Here's how the part is built. I have some questions about the finished solid (model axes, mm). A direction names the side the tool comes from. Give positions to 0.01 mm unless a question says otherwise; leave off trailing zeros. Write each loop counter-clockwise with the first axis right and the second up, starting at its lowest first coordinate (ties: lowest second). Pieces come first, ordered by that corner, then holes. Notation, with made-up numbers: (87.25, 11.25) -> (111.25, 11.25) arc R35 cw to (111.25, 50.25) -> close; hole circle Ø2 at (-26, 43). An arc over 180 degrees is marked (long way). Put each result on its own line as item: value. Start each with the question number.
from build123d import *

# Parameters (mm, degrees)
RESSALTO_EXTRUS_O1_DEPTH = 10
ESBO_O2_R                = 2.55
CORTE_EXTRUS_O1_DEPTH    = 10
ESBO_O4_R                = 19.5
CORTE_EXTRUS_O3_DEPTH    = 10
ESBO_O5_W                = 20
ESBO_O5_H                = 10
CORTE_EXTRUS_O4_DEPTH    = 30
ESBO_O6_R                = 1.75
CORTE_EXTRUS_O5_DEPTH    = 10
ESBO_O7_R                = 6
ESBO_O7_R_2              = 1.75
RESSALTO_EXTRUS_O2_DEPTH = 10
ESBO_O9_R                = 5
CORTE_EXTRUS_O6_DEPTH    = 4
ESBO_O10_R               = 3.5
CORTE_EXTRUS_O7_DEPTH    = 4


with BuildPart() as part:
    # Esboço1 → Ressalto-extrusão1 (new body)
    with BuildSketch(Plane.XY):
        with BuildLine():
            Line((25, -32.950849719), (-25, -32.950849719))
            ThreePointArc((-25, -32.950849719), (-28.535533906, -31.486383625), (-30, -27.950849719))
            Line((-30, -27.950849719), (-30, 27.950849719))
            ThreePointArc((-30, 27.950849719), (-28.535533906, 31.486383625), (-25, 32.950849719))
            Line((-25, 32.950849719), (25, 32.950849719))
            ThreePointArc((25, 32.950849719), (28.535533906, 31.486383625), (30, 27.950849719))
            Line((30, 27.950849719), (30, -27.950849719))
            ThreePointArc((30, -27.950849719), (28.535533906, -31.486383625), (25, -32.950849719))
        make_face()
    extrude(amount=RESSALTO_EXTRUS_O1_DEPTH)

    # Esboço2 → Corte-extrusão1 (cut)
    with BuildSketch(Plane.XY.offset(10)):
        with Locations((-23.57, 23.57)):
            Circle(ESBO_O2_R)
        with Locations((23.57, 23.57)):
            Circle(ESBO_O2_R)
        with Locations((23.57, -23.57)):
            Circle(ESBO_O2_R)
        with Locations((-23.57, -23.57)):
            Circle(ESBO_O2_R)
    extrude(amount=-CORTE_EXTRUS_O1_DEPTH, mode=Mode.SUBTRACT)

    # Esboço4 → Corte-extrusão3 (cut)
    with BuildSketch(Plane.XY.offset(10)):
        Circle(ESBO_O4_R)
    extrude(amount=-CORTE_EXTRUS_O3_DEPTH, mode=Mode.SUBTRACT)

    # Esboço5 → Corte-extrusão4 (cut)
    with BuildSketch(Plane.XZ.offset(32.950849719)):
        with Locations((0, 5)):
            Rectangle(ESBO_O5_W, ESBO_O5_H)
    extrude(amount=-CORTE_EXTRUS_O4_DEPTH, mode=Mode.SUBTRACT)

    # Esboço6 → Corte-extrusão5 (cut)
    with BuildSketch(Plane(origin=(0, 0, 0), x_dir=(-1, 0, 0), z_dir=(0, 0, -1))):
        with Locations((17.5, 30)):
            Circle(ESBO_O6_R)
        with Locations((-17.5, 30)):
            Circle(ESBO_O6_R)
        with Locations((-17.5, -30)):
            Circle(ESBO_O6_R)
        with Locations((17.5, -30)):
            Circle(ESBO_O6_R)
    extrude(amount=-CORTE_EXTRUS_O5_DEPTH, mode=Mode.SUBTRACT)

    # Esboço7 → Ressalto-extrusão2 (add)
    # profile 1 of 4: a face of its own
    with BuildSketch(Plane(origin=(0, 0, 0), x_dir=(-1, 0, 0), z_dir=(0, 0, -1))):
        with Locations((17.5, -30)):
            Circle(ESBO_O7_R)
        with Locations((17.5, -30)):
            Circle(ESBO_O7_R_2, mode=Mode.SUBTRACT)
    # profile 2 of 4: a face of its own
    with BuildSketch(Plane(origin=(0, 0, 0), x_dir=(-1, 0, 0), z_dir=(0, 0, -1))):
        with Locations((-17.5, -30)):
            Circle(ESBO_O7_R)
        with Locations((-17.5, -30)):
            Circle(ESBO_O7_R_2, mode=Mode.SUBTRACT)
    # profile 3 of 4: a face of its own
    with BuildSketch(Plane(origin=(0, 0, 0), x_dir=(-1, 0, 0), z_dir=(0, 0, -1))):
        with Locations((-17.5, 30)):
            Circle(ESBO_O7_R)
        with Locations((-17.5, 30)):
            Circle(ESBO_O7_R_2, mode=Mode.SUBTRACT)
    # profile 4 of 4: a face of its own
    with BuildSketch(Plane(origin=(0, 0, 0), x_dir=(-1, 0, 0), z_dir=(0, 0, -1))):
        with Locations((17.5, 30)):
            Circle(ESBO_O7_R)
        with Locations((17.5, 30)):
            Circle(ESBO_O7_R_2, mode=Mode.SUBTRACT)
    extrude(amount=-RESSALTO_EXTRUS_O2_DEPTH)

    # Esboço9 → Corte-extrusão6 (cut)
    with BuildSketch(Plane.XY.offset(10)):
        with Locations((23.57, 23.57)):
            Circle(ESBO_O9_R)
        with Locations((-23.57, 23.57)):
            Circle(ESBO_O9_R)
        with Locations((23.57, -23.57)):
            Circle(ESBO_O9_R)
        with Locations((-23.57, -23.57)):
            Circle(ESBO_O9_R)
    extrude(amount=-CORTE_EXTRUS_O6_DEPTH, mode=Mode.SUBTRACT)

    # Esboço10 → Corte-extrusão7 (cut)
    with BuildSketch(Plane(origin=(0, 0, 0), x_dir=(-1, 0, 0), z_dir=(0, 0, -1))):
        with Locations((-17.5, -30)):
            Circle(ESBO_O10_R)
        with Locations((17.5, -30)):
            Circle(ESBO_O10_R)
        with Locations((17.5, 30)):
            Circle(ESBO_O10_R)
        with Locations((-17.5, 30)):
            Circle(ESBO_O10_R)
    extrude(amount=-CORTE_EXTRUS_O7_DEPTH, mode=Mode.SUBTRACT)


solid = part.part
1) Thinking about a two-plate mould opening in Y: for faces 1 (the cylindrical face through (18.89, -31.06, 6.96)), 2 (the flat face through (-24, 32.951, 5)), 3 (the cylindrical face through (-17.4, -36, 4.9)), which applies, released by +Y, released by -Y, zero draft, split by the parting line, or undercut?
2) I want a section at D-D, the plane y = -23.57. Write out the boundary of the cut face in (x, z).
3) Which directions (+Z, -Z, +X, -X, +Y, -Y) give clear straight access to the entire face, cutting with the end or side of a thin tool? Please do faces 4 (the cylindrical face through (22.919, 28.527, 8.028)), 5 (the flat face through (-24, -32.951, 5)), 6 (the cylindrical face through (17.4, 36, 4.9)), 7 (the flat face through (-18, 32, 4)).
4) I'm going to push flat-ended pins straight in: pin 1 Ø5.5 at (x, y) = (-17.5, -30) entering from -Z; pin 2 Ø3 at (x, z) = (22, 3.5) entering from +Y; pin 3 Ø2 at (x, z) = (-11, 6.5) entering from -Y; pin 4 Ø3 at (x, y) = (17.5, -30) entering from -Z. Where does each tip first touch, or does it pass through?
5) I want a section at C-C, the plane z = 5. State how many separate pieces and enclosed holes the cut face has, and give its area (3 significant figures).
6) I need wall thicknesses on probe 1 along X at (y, z) = (23.5, 4); probe 2 along Y at (x, z) = (-24, 7.5); probe 3 along X at (y, z) = (-22.5, 4.75). Which ranges of each line are inside material? Lowest first, please.
7) I want a section at A-A, the plane y = 23.57. Write out the boundary of the cut face in (x, z).
8) I want a section at B-B, the plane x = -23.57. Write out the boundary of the cut face in (y, z).
Established:
1. face 1: undercut
1. face 2: released by +Y
1. face 3: released by -Y
2. outline: (-30, 0) -> (-26.12, 0) -> (-26.12, 6) -> (-28.57, 6) -> (-28.57, 10) -> (-30, 10) -> close; (-21.02, 0) -> (-10, 0) -> (-10, 10) -> (-18.57, 10) -> (-18.57, 6) -> (-21.02, 6) -> close; (10, 0) -> (21.02, 0) -> (21.02, 6) -> (18.57, 6) -> (18.57, 10) -> (10, 10) -> close; (26.12, 0) -> (30, 0) -> (30, 10) -> (28.57, 10) -> (28.57, 6) -> (26.12, 6) -> close
3. face 4: +Z
3. face 5: +Z, -Z, -X, -Y
3. face 6: +Z, -Z, +Y
3. face 7: -Z
4. pin 1: stops at z = 4
4. pin 2: stops at y = 35.2
4. pin 3: stops at y = -32.95
4. pin 4: passes through
5. separate pieces: 1
5. enclosed holes: 8
5. area: 2,420 mm2
6. probe 1: x = -30 to -26.12, -21.02 to 21.02, 26.12 to 30
6. probe 2: y = -32.95 to -28.55, -18.59 to 18.59, 28.55 to 32.95
6. probe 3: x = -30 to -25.88, -21.26 to -10, 10 to 21.26, 25.88 to 30
7. outline: (-30, 0) -> (-26.12, 0) -> (-26.12, 6) -> (-28.57, 6) -> (-28.57, 10) -> (-30, 10) -> close; (-21.02, 0) -> (21.02, 0) -> (21.02, 6) -> (18.57, 6) -> (18.57, 10) -> (-18.57, 10) -> (-18.57, 6) -> (-21.02, 6) -> close; (26.12, 0) -> (30, 0) -> (30, 10) -> (28.57, 10) -> (28.57, 6) -> (26.12, 6) -> close
8. outline: (-32.95, 0) -> (-26.12, 0) -> (-26.12, 6) -> (-28.57, 6) -> (-28.57, 10) -> (-32.95, 10) -> close; (-21.02, 0) -> (21.02, 0) -> (21.02, 6) -> (18.57, 6) -> (18.57, 10) -> (-18.57, 10) -> (-18.57, 6) -> (-21.02, 6) -> close; (26.12, 0) -> (32.95, 0) -> (32.95, 10) -> (28.57, 10) -> (28.57, 6) -> (26.12, 6) -> close
